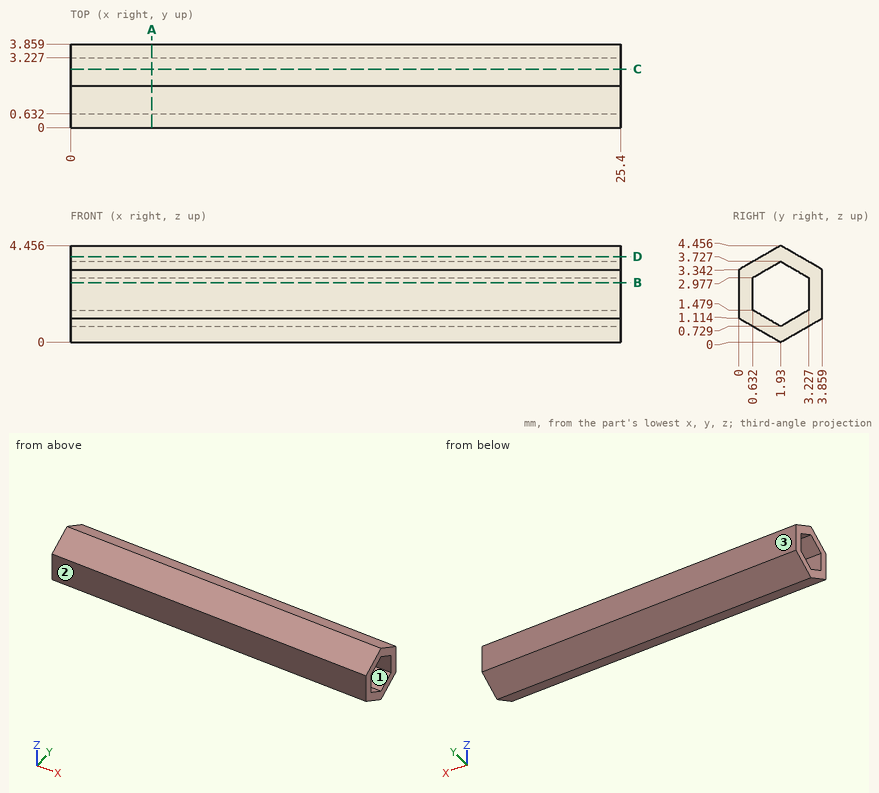
Part print with two shaded views. Sizes in mm from the minimum x, y, z corner. Round coordinates to 2 decimals unless told otherwise and drop trailing zeros. Order: outer loops, then holes, each group sorted by start corner. A loop starts at its lowest first (then second) coordinate and runs counter-clockwise, first axis right, second up.
(1) Band-saw the part on B-B (z = 2.75). List the corners of the cut face in (x, y).
(2) Drill centre lines: line 1 (Y direction, x = 1.25, z = 2.15); line 2 (Y direction, x = 24.25, z = 3.3) (1 decimal); line 3 (Z direction, x = 17.75, y = 1.7) (1 decimal). Where is each one in solid material? Low to high.
(3) Band-saw the part on A-A (x = 3.75). List the corners of the cut face in (y, z) (1 decimal).
(4) Pull direction Y, two halves, no side cores. Call the marked faces 1, 2 and 3: released by +Y, released by -Y, zero draft, split by the parting line, or undercut.
(5) Band-saw the part on D-D (z = 3.95). List the corners of the cut face in (x, y) (1 decimal).
(6) Band-saw the part on C-C (y = 2.7). List the corners of the cut face in (x, z) (1 decimal).
Verdict:
1. outline: (0, 0) - (25.4, 0) - (25.4, 0.63) - (0, 0.63) - close; (0, 3.23) - (25.4, 3.23) - (25.4, 3.86) - (0, 3.86) - close
2. line 1: y = 0 to 0.63, 3.23 to 3.86
2. line 2: y = 0 to 1.2, 2.7 to 3.9
2. line 3: z = 0.1 to 0.9, 3.6 to 4.3
3. outline: (0, 1.1) - (1.9, 0) - (3.9, 1.1) - (3.9, 3.3) - (1.9, 4.5) - (0, 3.3) - close; hole (0.6, 1.5) - (1.9, 0.7) - (3.2, 1.5) - (3.2, 3) - (1.9, 3.7) - (0.6, 3) - close
4. face 1: undercut
4. face 2: released by -Y
4. face 3: released by +Y
5. outline: (0, 1.1) - (25.4, 1.1) - (25.4, 2.8) - (0, 2.8) - close
6. outline: (0, 0.4) - (25.4, 0.4) - (25.4, 1.2) - (0, 1.2) - close; (0, 3.3) - (25.4, 3.3) - (25.4, 4) - (0, 4) - close
